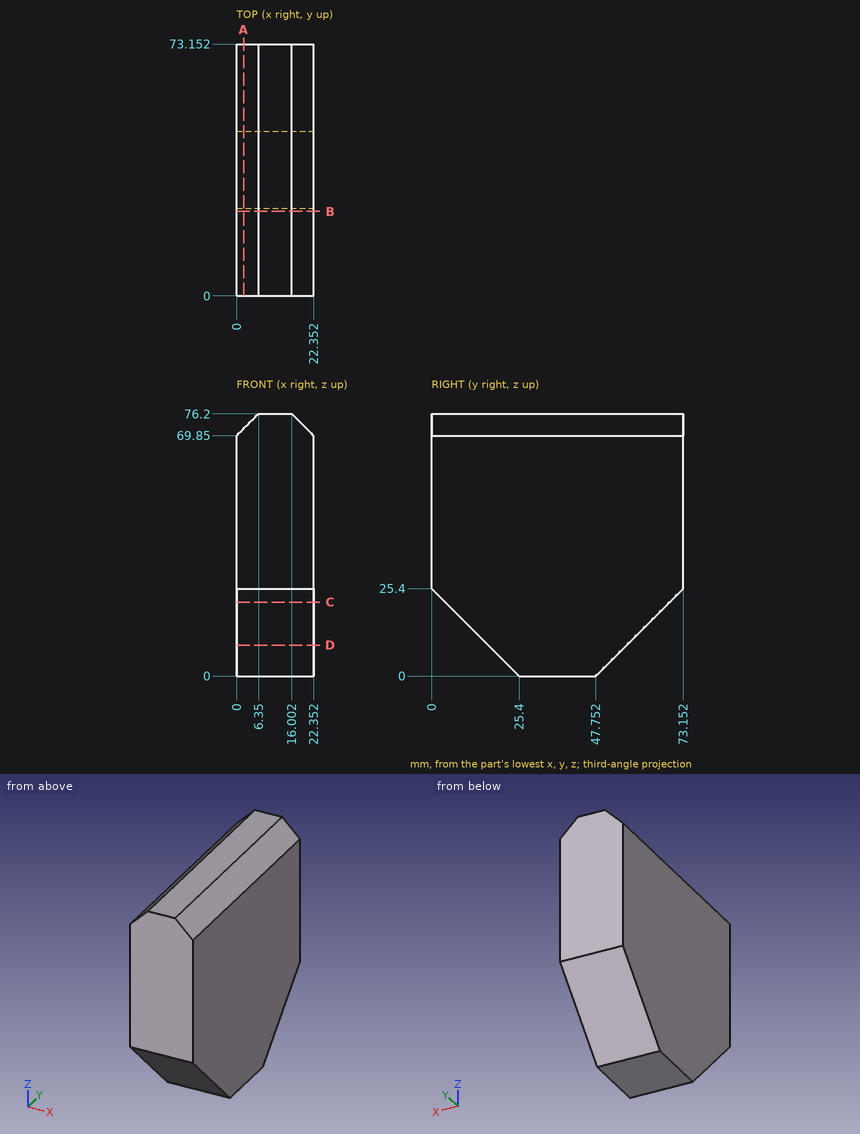
The figure shows three views and two pictorial views of one solid part (mm, origin at its lowest corner). Answer the questions. Round coordinates to 2 decimals unless told otherwise and drop trailing zeros. Order: outer loops, then holes, each group sorted by start corner. A loop starts at its lowest first (then second) coordinate and runs counter-clockwise, first axis right, second up. Notation, with made-up numbers: (-30, 50) - (15, 50) arc R27 ccw to (15, 84) - close; hole circle Ø8 at (31.25, 61.25). An arc over 180 degrees is marked (long way). Write item = value, one per line. Start each with the question number.
1) Given pin 1 (12 mm diameter, centred on x = 9, z = 14, fed in from +Y); pin 2 (12 mm diameter, centred on x = 15, z = 11.5, fed in from -Y); pin 3 (6 mm diameter, centred on x = 10.5, y = 12, fed in from -Z), each flat-ended and moving along its own axis, determine where each tip first touches the part or whether it passes through.
2) Section B-B, the plane y = 24.5 is taken. Write down the section's boundary in (x, z), plus the area to 3 significant figures.
3) Section A-A, the plane x = 2 is taken. Write down the section's boundary in (y, z).
4) Section C-C, the plane z = 21.5 is taken. Write down the section's boundary in (x, y).
5) Section D-D, the plane z = 9 is taken. Write down the section's boundary in (x, y).
6) Straight lines are drawn through the part: L1, parallel to Y at x = 15.75, z = 23; L2, parallel to Z at x = 15.5, y = 62.5; L3, parallel to Z at x = 21.75, y = 47.5. For each, find the intervals that lie inside material, in ascending order.
Results list:
q1.pin_1 = 67.75
q1.pin_2 = 7.9
q1.pin_3 = 10.4
q2.outline = (0, 0.9) - (22.35, 0.9) - (22.35, 69.85) - (16, 76.2) - (6.35, 76.2) - (0, 69.85) - close
q2.area = 1,640 mm^2
q3.outline = (0, 25.4) - (25.4, 0) - (47.75, 0) - (73.15, 25.4) - (73.15, 71.85) - (0, 71.85) - close
q4.outline = (0, 3.9) - (22.35, 3.9) - (22.35, 69.25) - (0, 69.25) - close
q5.outline = (0, 16.4) - (22.35, 16.4) - (22.35, 56.75) - (0, 56.75) - close
q6.L1 = 2.4 to 70.75
q6.L2 = 14.75 to 76.2
q6.L3 = 0 to 70.45
